Geometry check sheet. Reference: the model listing, model coordinates, mm. A direction names the side the tool comes from. Round coordinates to 2 decimals unless told otherwise and drop trailing zeros. Order: outer loops, then holes, each group sorted by start corner. A loop starts at its lowest first (then second) coordinate and runs counter-clockwise, first axis right, second up.
(1) Set-up check for faces 1 (the face through (-8, 15, 0)), 2 (the face through (-11, -8, 5)), 3 (the face through (-4.86, 18.83, 2.84)), 4 (the face through (0, 38, 2)), 5 (the face through (0, -7, 2)): record each of +Z, -Z, +X, -X, +Y, -Y from which the full face is reachable in a straight line by a thin tool's end or side.
(2) Sectioned sample at C-C (z = 15). Record the boundary of the cut face in (x, y).
(3) Sectioned sample at A-A (y = -7.5). Record the boundary of the cut face in (x, z), plus the area to 3 significant figures.
(4) Sectioned sample at B-B (x = -7.5). Record the boundary of the cut face in (y, z).
(5) Release check for a two-part mould opening along Y. For faces 6 (the face through (-8, 45, 2)), 7 (the face through (-8, 34, 5)), 8 (the face through (-6.96, 35.06, 2.46)) record: +Y half, -Y half, draft (parallel to the pull), parting line (faces both ways), or undercut.
(6) Sectioned sample at D-D (y = 15). Record the boundary of the cut face in (x, z).
(7) Go/stop test with flat-tipped pins: pin 1 (4 mm diameter, centred on y = 31.5, z = 10, fed in from -X); pin 2 (10 mm diameter, centred on x = -2, z = 18.5, fed in from -Y); pin 3 (6 mm diameter, centred on x = -7.5, y = -7.5, fed in from -Z); pin 4 (7.5 mm diameter, centred on y = 19, z = -6.5, fed in from -X). Record where each tip stops, or that it passes through.
(8) Material ranges on line 1 along Y through (x, z) = (-7.5, 1.5); line 2 along Y through (x, z) = (-8.25, 15); line 3 along Z through (x, y) = (-4, 14.5), recorded low to high.
from build123d import *

# Parameters (mm, degrees)
SKETCH1_W           = 30
SKETCH1_H           = 15
BOSS_EXTRUDE1_DEPTH = 30
SKETCH2_W           = 30
SKETCH2_H           = 45
BOSS_EXTRUDE2_DEPTH = 5
SKETCH5_R           = 2.5
CUT_EXTRUDE2_DEPTH  = 47.904157598
SKETCH3_R           = 12.75
CUT_EXTRUDE3_DEPTH  = 47.904157598
SKETCH8_W           = 15
SKETCH8_H           = 15
SKETCH8_R           = 2.5
BOSS_EXTRUDE4_DEPTH = 5


with BuildPart() as part:
    # Sketch1 → Boss-Extrude1 (new body)
    with BuildSketch(Plane(origin=(0, 0, 0), x_dir=(0, 1, 0), z_dir=(0, 0, 1))):
        with Locations((15, 7.5)):
            Rectangle(SKETCH1_W, SKETCH1_H)
    extrude(amount=BOSS_EXTRUDE1_DEPTH)

    # Sketch2 → Boss-Extrude2 (add)
    with BuildSketch(Plane.YZ):
        with Locations((15, 7.5)):
            Rectangle(SKETCH2_W, SKETCH2_H)
    extrude(amount=BOSS_EXTRUDE2_DEPTH)

    # Sketch5 → Cut-Extrude2 (cut, through all)
    with BuildSketch(Plane.YZ.offset(5)):
        with Locations(Location((15, -7.5, 0), (0, 0, 270))):
            Circle(SKETCH5_R)
    extrude(amount=-CUT_EXTRUDE2_DEPTH, mode=Mode.SUBTRACT)

    # Sketch3 → Cut-Extrude3 (cut, through all)
    with BuildSketch(Plane.YZ.offset(5)):
        with Locations(Location((15, 15, 0), (0, 0, 270))):
            Circle(SKETCH3_R)
    extrude(amount=-CUT_EXTRUDE3_DEPTH, mode=Mode.SUBTRACT)

    # Sketch8 → Boss-Extrude4 (add)
    # profile 1 of 2: a face of its own
    with BuildSketch(Plane(origin=(0, 0, 0), x_dir=(1, 0, 0), z_dir=(0, 0, -1))):
        with Locations((-7.5, -37.5)):
            Rectangle(SKETCH8_W, SKETCH8_H)
        with Locations(Location((-7.5, -37.5, 0), (0, 0, 180))):
            Circle(SKETCH8_R, mode=Mode.SUBTRACT)
    # profile 2 of 2: a face of its own
    with BuildSketch(Plane(origin=(0, 0, 0), x_dir=(1, 0, 0), z_dir=(0, 0, -1))):
        with Locations((-7.5, 7.5)):
            Rectangle(SKETCH8_W, SKETCH8_H)
        with Locations(Location((-7.5, 7.5, 0), (0, 0, 180))):
            Circle(SKETCH8_R, mode=Mode.SUBTRACT)
    extrude(amount=-BOSS_EXTRUDE4_DEPTH)


solid = part.part
Answer below:
1. face 1: -Z, -X, +Y, -Y
1. face 2: +Z, +X, -X, -Y
1. face 3: +X, -X
1. face 4: +Z, -Z, +X, +Y
1. face 5: +Z, -Z, +X, -Y
2. outline: (-15, 0) - (5, 0) - (5, 2.25) - (-15, 2.25) - close; (-15, 27.75) - (5, 27.75) - (5, 30) - (-15, 30) - close
3. outline: (-15, 0) - (-10, 0) - (-10, 5) - (-15, 5) - close; (-5, 0) - (0, 0) - (0, 5) - (-5, 5) - close
3. area: 50.0 mm2
4. outline: (-15, 0) - (-10, 0) - (-10, 5) - (-15, 5) - close; (-5, 0) - (35, 0) - (35, 5) - (30, 5) - (30, 30) - (0, 30) - (0, 5) - (-5, 5) - close; (40, 0) - (45, 0) - (45, 5) - (40, 5) - close; hole circle Ø25.5 at (15, 15)
5. face 6: +Y half
5. face 7: draft
5. face 8: undercut
6. outline: (-15, 0) - (0, 0) - (0, -5) - (5, -5) - (5, 2.25) - (-15, 2.25) - close; (-15, 27.75) - (5, 27.75) - (5, 30) - (-15, 30) - close; (0, -15) - (5, -15) - (5, -10) - (0, -10) - close
7. pin 1: stops at x = -15
7. pin 2: stops at y = 0
7. pin 3: stops at z = 0
7. pin 4: stops at x = 0
8. line 1: y = -15 to -10, -5 to 35, 40 to 45
8. line 2: y = 0 to 2.25, 27.75 to 30
8. line 3: z = 0 to 2.26, 27.74 to 30
